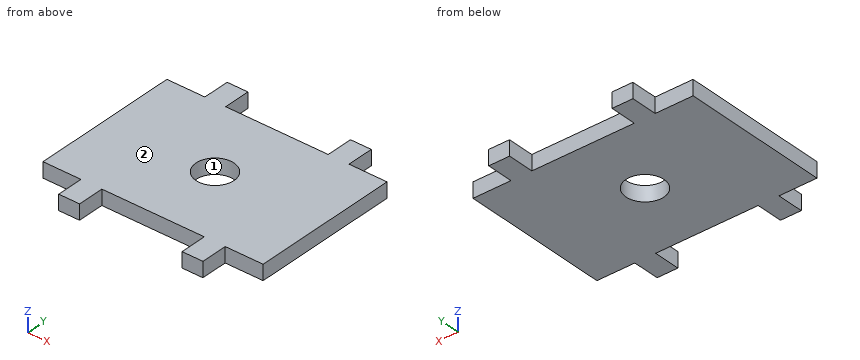
Autodesk Inventor part; units mm, degrees
ref_plane "YZ Plane" through (0, 0, 0) normal (1, 0, 0) x (0, 1, 0)
ref_plane "XZ Plane" through (0, 0, 0) normal (0, 1, 0) x (-1, 0, 0)
ref_plane "XY Plane" through (0, 0, 0) normal (0, 0, 1) x (1, 0, 0)
sketch "Эскиз1" plane through (0, 0, 0) normal (0, 0, 1) x (1, 0, 0)
  line L0 (14.5, 9.75) -> (14.5, -9.75)
  line L1 (-14.5, -9.75) -> (-14.5, 9.75)
  line L2 (9.5, 9.75) -> (9.5, 13.25)
  line L3 (9.5, 13.25) -> (6.75, 13.25)
  line L4 (6.75, 13.25) -> (6.75, 9.75)
  line L5 (-9.5, 9.75) -> (-9.5, 13.25)
  line L6 (-9.5, 13.25) -> (-6.75, 13.25)
  line L7 (-6.75, 13.25) -> (-6.75, 9.75)
  line L8 (9.5, -9.75) -> (9.5, -13.25)
  line L9 (9.5, -13.25) -> (6.75, -13.25)
  line L10 (6.75, -13.25) -> (6.75, -9.75)
  line L11 (-6.75, -13.25) -> (-6.75, -9.75)
  line L12 (-9.5, -13.25) -> (-6.75, -13.25)
  line L13 (-9.5, -9.75) -> (-9.5, -13.25)
  line L14 (14.5, 9.75) -> (9.5, 9.75)
  line L15 (6.75, 9.75) -> (-6.75, 9.75)
  line L16 (-9.5, 9.75) -> (-14.5, 9.75)
  line L17 (-9.5, -9.75) -> (-14.5, -9.75)
  line L18 (14.5, -9.75) -> (9.5, -9.75)
  line L19 (6.75, -9.75) -> (-6.75, -9.75)
  circle A0 centre (0, 0) radius 2.5
  point P0 (-14.5, 0)
  dimension "d0" = 29
  dimension "d1" = 19.5
  dimension "d2" = 5
  dimension "d3" = 3.5
  dimension "d4" = 2.75
  dimension "d7" = 5
extrude "Выдавливание1" add sketch "Эскиз1" along normal blind 2
properties part number "Крепеж колеса"
Geometry: final body of the model. Coordinates: model frame, mm. Face numbers are marked on the shaded views. Give positions to 0.01 mm unless a question says otherwise; leave off trailing zeros. Write each loop counter-clockwise with the first axis right and the second up, starting at its lowest first coordinate (ties: lowest second). Pieces come first, ordered by that corner, then holes. Notation, with made-up numbers: (54, 43) -> (86, 43) arc R12 ccw to (86, 61) -> close; hole circle Ø9 at (61.5, -29). An arc over 180 degrees is marked (long way). Answer in a Markdown table with one row per item.
(1) Draft query along X for the marked faces 1 and 2. Return one class per face: +X half, -X half, draft (parallel to the pull), parting line (faces both ways), or undercut.
Answers below:
| item | result |
|---|---|
| face 1 | undercut |
| face 2 | draft |
(2) Section query B-B on z = 1.6. Return loops of the section in (x, y), then the cut area to 3 significant figures.
Answers below:
| item | result |
|---|---|
| outline | (-14.5, -9.75) -> (-9.5, -9.75) -> (-9.5, -13.25) -> (-6.75, -13.25) -> (-6.75, -9.75) -> (6.75, -9.75) -> (6.75, -13.25) -> (9.5, -13.25) -> (9.5, -9.75) -> (14.5, -9.75) -> (14.5, 9.75) -> (9.5, 9.75) -> (9.5, 13.25) -> (6.75, 13.25) -> (6.75, 9.75) -> (-6.75, 9.75) -> (-6.75, 13.25) -> (-9.5, 13.25) -> (-9.5, 9.75) -> (-14.5, 9.75) -> close; hole circle Ø5 at (0, 0) |
| area | 584 mm^2 |
(3) Ray query, line 1 along Y through (x, z) = (0, 1.55); line 2 along X through (y, z) = (-10.25, 0.2); line 3 along Y through (x, z) = (4.5, 1.4). Return the intervals inside material, ascending. Write a range as [from, to].
Answers below:
| item | result |
|---|---|
| line 1 | [-9.75, -2.5], [2.5, 9.75] |
| line 2 | [-9.5, -6.75], [6.75, 9.5] |
| line 3 | [-9.75, 9.75] |
(4) Section query D-D on x = -6. Return loops of the section in (y, z).
Answers below:
| item | result |
|---|---|
| outline | (-9.75, 0) -> (9.75, 0) -> (9.75, 2) -> (-9.75, 2) -> close |
(5) Section query C-C on x = 0. Return loops of the section in (y, z).
Answers below:
| item | result |
|---|---|
| outline | (-9.75, 0) -> (-2.5, 0) -> (-2.5, 2) -> (-9.75, 2) -> close; (2.5, 0) -> (9.75, 0) -> (9.75, 2) -> (2.5, 2) -> close |
(6) Section query A-A on y = 0. Return loops of the section in (x, z), then the cut area to 3 significant figures.
Answers below:
| item | result |
|---|---|
| outline | (-14.5, 0) -> (-2.5, 0) -> (-2.5, 2) -> (-14.5, 2) -> close; (2.5, 0) -> (14.5, 0) -> (14.5, 2) -> (2.5, 2) -> close |
| area | 48.0 mm^2 |
(7) Pin query (flat end, axial travel): pin 1 (1 mm diameter, centred on x = -11, z = 1, fed in from +Y); pin 2 (1 mm diameter, centred on y = -11, z = 1.5, fed in from -X); pin 3 (1 mm diameter, centred on y = -12, z = 1.5, fed in from +X). Return the tip coordinate at first contact, or that it passes through.
Answers below:
| item | result |
|---|---|
| pin 1 | y = 9.75 |
| pin 2 | x = -9.5 |
| pin 3 | x = 9.5 |
